```python
from build123d import *

# Parameters (mm, degrees)
PAD_DEPTH         = 28
CYLINDER_R        = 2.5
CYLINDER_DEPTH    = 6
CYLINDER001_R     = 2.5
CYLINDER001_DEPTH = 6
CYLINDER002_R     = 2.5
CYLINDER002_DEPTH = 6
CYLINDER003_R     = 2.5
CYLINDER003_DEPTH = 6


with BuildPart() as part:
    # Sketch → Pad (new body)
    with BuildSketch(Plane.XZ):
        Polygon((-60, 0), (-60, -60), (60, -60), (60, 60), (-60, 60), align=None)
    extrude(amount=PAD_DEPTH)

    # Cylinder → Cylinder (join)
    with BuildSketch(Plane(origin=(-52.5, 6, 52.5), x_dir=(1, 0, 0), z_dir=(0, -1, 0))):
        Circle(CYLINDER_R)
    extrude(amount=CYLINDER_DEPTH)

    # Cylinder001 → Cylinder001 (join)
    with BuildSketch(Plane(origin=(52.5, 6, 52.5), x_dir=(1, 0, 0), z_dir=(0, -1, 0))):
        Circle(CYLINDER001_R)
    extrude(amount=CYLINDER001_DEPTH)

    # Cylinder002 → Cylinder002 (join)
    with BuildSketch(Plane(origin=(52.5, 6, -52.5), x_dir=(1, 0, 0), z_dir=(0, -1, 0))):
        Circle(CYLINDER002_R)
    extrude(amount=CYLINDER002_DEPTH)

    # Cylinder003 → Cylinder003 (join)
    with BuildSketch(Plane(origin=(-52.5, 6, -52.5), x_dir=(1, 0, 0), z_dir=(0, -1, 0))):
        Circle(CYLINDER003_R)
    extrude(amount=CYLINDER003_DEPTH)


solid = part.part
```
Geometry check sheet. Reference: the model listing, model coordinates, mm. A direction names the side the tool comes from. Coordinates: 2 decimals unless noted, no trailing zeros. Write each loop counter-clockwise with the first axis right and the second up, starting at its lowest first coordinate (ties: lowest second). Pieces come first, ordered by that corner, then holes. Notation, with made-up numbers: M 82,-38.75 L 126,-38.75 A26 cw 126,-16.75 Z; hole C -3.75,69 d6. An arc over 180 degrees is marked long. One line per item, written item: value. Start each with the question number.
(1) Depth check by flat-ended pin: pin 1 (12 mm diameter, centred on x = -42, z = -31.5, fed in from +Y). Enter the tip coordinate at first touch or a pass-through.
(2) Sectioned sample at B-B, the plane z = 52.5. Enter the section's corners in (x, y).
(3) Scan lines: line 1 along Y through (x, z) = (-29.5, -52.5); line 2 along Z through (x, y) = (50.5, 1). Record each from-to range of solid material in increasing order. Write a range as [from, to].
(4) Sectioned sample at C-C, the plane z = 3. Enter the section's corners in (x, y), and give its area (3 significant figures).
(5) Tool access check on faces 1 (the face through (1, -14, 60)), 2 (the face through (-1, 0, 1)). Record the directions out of +Z, -Z, +X, -X, +Y, -Y that give a thin tool (end or side, any length) a straight path to the whole face; none if there is none.
(6) Sectioned sample at A-A, the plane x = -52.5. Enter the section's corners in (y, z), and give its area (3 significant figures).
Filled sheet:
1. pin 1: y = 0
2. outline: M -60,-28 L 60,-28 L 60,0 L 55,0 L 55,6 L 50,6 L 50,0 L -50,0 L -50,6 L -55,6 L -55,0 L -60,0 Z
3. line 1: [-28, 0]
3. line 2: [-54, -51], [51, 54]
4. outline: M -60,-28 L 60,-28 L 60,0 L -60,0 Z
4. area: 3,360 mm²
5. face 1: +Z, +X, -X, +Y, -Y
5. face 2: +Y
6. outline: M -28,-60 L 0,-60 L 0,-55 L 6,-55 L 6,-50 L 0,-50 L 0,50 L 6,50 L 6,55 L 0,55 L 0,60 L -28,60 Z
6. area: 3,420 mm²
